The model under review builds one solid part; all positions refer to its coordinate system, in mm. Coordinates: 2 decimals unless noted, no trailing zeros. Loops run counter-clockwise (first coordinate to the right, second up) from the corner with the lowest first, then second, coordinate; pieces in that order, holes last. Notation, with made-up numbers: (57.5, 89.25) - (109.5, 89.25) arc R19 ccw to (109.5, 124.25) - close; hole circle Ø7 at (6, -39.75). An arc over 180 degrees is marked (long way). Use a Markdown table: item, result. Add a question column.
1) Add section A-A, the plane x = 172.5. Give the boundary of the cut face in (y, z), and give its area (3 significant figures).
2) To check wall thickness, follow L1, parallel to Y at x = -451, z = 12.5; L2, parallel to X at y = 72, z = 7.75; L3, parallel to Z at x = 750, y = 0. State the ranges of each line that lie inside material, in increasing order. Write a range as [from, to].
3) Clearance check with a flat-ended pin moving along its axis: pin 1 (6 mm diameter, centred on x = 750, z = 12.5, fed in from +Y). State where the tip first meets the part, or that it passes through.
4) Add section B-B, the plane y = 199.5. Give the boundary of the cut face in (x, z).
5) Add section C-C, the plane z = 12.5. Give the number of separate pieces and of enclosed holes in the cut face, and give its area (3 significant figures).
```python
from build123d import *

# Parameters (mm, degrees)
F0_W     = 1900
F0_H     = 800
F1_DEPTH = 25
F2_R     = 5
F3_DEPTH = 800.001


with BuildPart() as f1:
    # F0 (on Top) → F1 (new body)
    with BuildSketch(Plane.XY):
        Rectangle(F0_W, F0_H)
        Polygon((20, 360), (910, 360), (910, 20), (910, -20), (910, -360), (20, -360), (-20, -360), (-910, -360), (-910, -20), (-910, 20), (-910, 360), (-20, 360), align=None, mode=Mode.SUBTRACT)
        Polygon((20, 20), (20, 360), (-20, 360), (-20, 20), (-910, 20), (-910, -20), (-20, -20), (-20, -360), (20, -360), (20, -20), (910, -20), (910, 20), align=None)
    extrude(amount=F1_DEPTH)

    # F2 (on face) → F3 (cut, through all)
    with BuildSketch(Plane.XZ.offset(400)):
        with Locations((750, 12.5)):
            Circle(F2_R)
        with Locations((-750, 12.5)):
            Circle(F2_R)
    extrude(amount=-F3_DEPTH, mode=Mode.SUBTRACT)


solid = f1.part
```
From the geometry:
| question | item | result |
|---|---|---|
| 1 | outline | (-400, 0) - (-360, 0) - (-360, 25) - (-400, 25) - close; (-20, 0) - (20, 0) - (20, 25) - (-20, 25) - close; (360, 0) - (400, 0) - (400, 25) - (360, 25) - close |
| 1 | area | 3,000 mm^2 |
| 2 | L1 | y = [-400, -360], [-20, 20], [360, 400] |
| 2 | L2 | x = [-950, -910], [-20, 20], [910, 950] |
| 2 | L3 | z = [0, 7.5], [17.5, 25] |
| 3 | pin 1 | passes through |
| 4 | outline | (-950, 0) - (-910, 0) - (-910, 25) - (-950, 25) - close; (-20, 0) - (20, 0) - (20, 25) - (-20, 25) - close; (910, 0) - (950, 0) - (950, 25) - (910, 25) - close |
| 5 | separate pieces | 3 |
| 5 | enclosed holes | 0 |
| 5 | area | 307,000 mm^2 |
